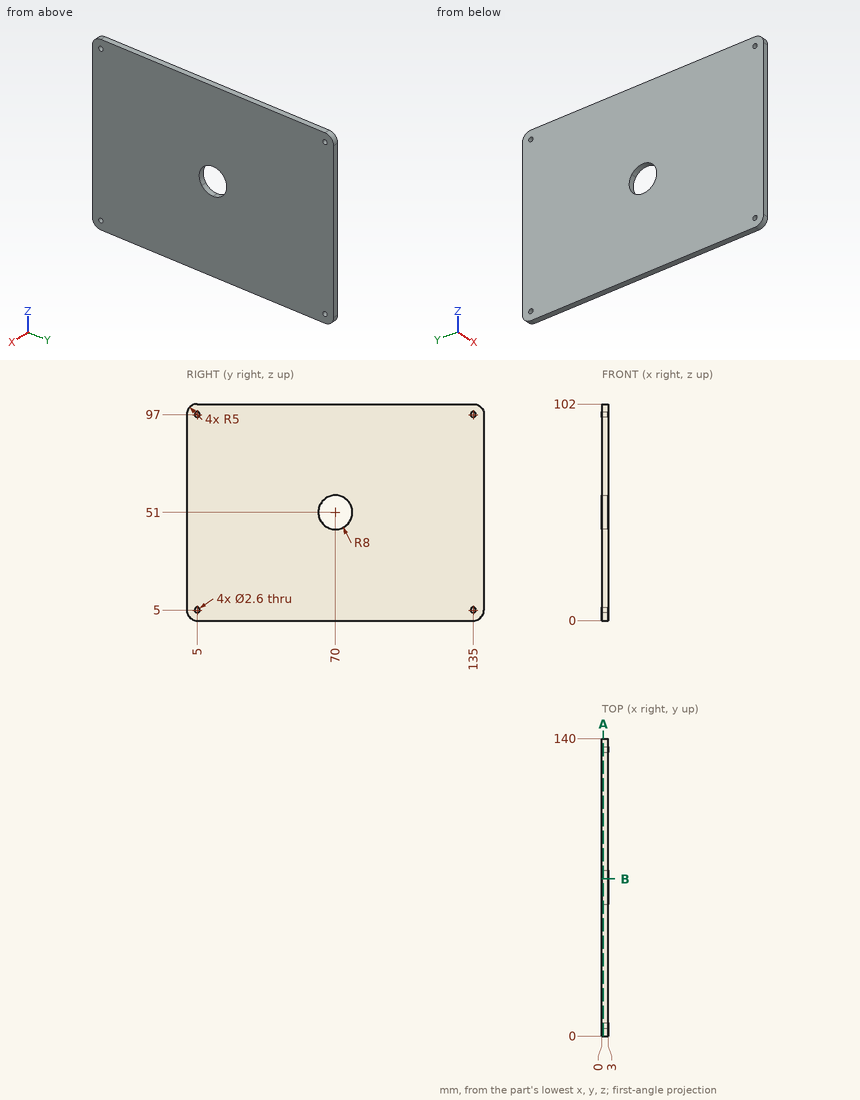
Geometry check sheet. Reference: drawing and pictorial views, mm from the part's lowest x, y, z. Round coordinates to 2 decimals unless told otherwise and drop trailing zeros. Loops run counter-clockwise (first coordinate to the right, second up) from the corner with the lowest first, then second, coordinate; pieces in that order, holes last. Notation, with made-up numbers: M 77.5,47 L 100.5,47 A29 ccw 100.5,80 Z; hole C 49.5,14 d9. An arc over 180 degrees is marked long. One line per item, written item: value.
(1) Thickness scan on line 1 (Z direction, x = 1.3, y = 5); line 2 (Y direction, x = 1.3, z = 5); line 3 (Z direction, x = 2.3, y = 69). Record the ranges inside material, lowest first.
Computed values:
line 1: z = 0 to 3.7, 6.3 to 95.7, 98.3 to 102
line 2: y = 0 to 3.7, 6.3 to 133.7, 136.3 to 140
line 3: z = 0 to 43.06, 58.94 to 102
(2) Depth check by flat-ended pin: pin 1 Ø3 at (y, z) = (135, 5) entering from +X; pin 2 Ø1.6 at (y, z) = (135, 97) entering from +X. Enter the tip coordinate at first touch or a pass-through.
Computed values:
pin 1: stops at x = 3
pin 2: passes through
(3) Sectioned sample at B-B, the plane y = 74. Record the cut outline in (x, z).
Computed values:
outline: M 0,0 L 3,0 L 3,44.07 L 0,44.07 Z; M 0,57.93 L 3,57.93 L 3,102 L 0,102 Z
(4) Sectioned sample at A-A, the plane x = 0.6. Record the cut outline in (y, z), then the cut area to 3 significant figures.
Computed values:
outline: M 0,5 A5 ccw 5,0 L 135,0 A5 ccw 140,5 L 140,97 A5 ccw 135,102 L 5,102 A5 ccw 0,97 Z; hole C 5,5 d2.6; hole C 5,97 d2.6; hole C 70,51 d16; hole C 135,5 d2.6; hole C 135,97 d2.6
area: 14,000 mm^2
